Part model, mm, in its own coordinate system. Face numbers are marked on the shaded views. A direction names the side the tool comes from. Round coordinates to 2 decimals unless told otherwise and drop trailing zeros. Loops run counter-clockwise (first coordinate to the right, second up) from the corner with the lowest first, then second, coordinate; pieces in that order, holes last. Notation, with made-up numbers: (-28.5, 19.5) -> (19.5, 19.5) arc R19 ccw to (19.5, 42.5) -> close; hole circle Ø9 at (0, 19). An arc over 180 degrees is marked (long way). Use a Markdown table: item, result. Add a question column.
Item 1: Cut at D-D, the plane x = -0.5. List the corners of the cut face in (y, z).
Item 2: Cut at B-B, the plane y = 8. List the corners of the cut face in (x, z), plus the area to 3 significant figures.
Item 3: Probe line 1 (X direction, y = 2.75, z = -5.15); line 2 (Z direction, x = 11.1, y = 2); line 3 (Z direction, x = -11.1, y = 6.75). List the from-to ranges inside material, lowest first. Write a range as [from, to].
Item 4: Cut at A-A, the plane x = 11.1. List the corners of the cut face in (y, z).
Item 5: Cut at C-C, the plane z = -5.15. List the corners of the cut face in (x, y).
Item 6: Flat gauge pins, fed straight in: pin 1 (2 mm diameter, centred on x = -6.5, z = -9.5, fed in from +Y); pin 2 (1.2 mm diameter, centred on x = -6, z = -9, fed in from -Y); pin 3 (2.5 mm diameter, centred on x = 19, y = 4.5, fed in from +Z); pin 4 (5 mm diameter, centred on x = 11.1, z = -5.15, fed in from -Y). Where does each tip first touch, or does it go through?
Item 7: Which spindle directions (+Z, -Z, +X, -X, +Y, -Y) get a long thin tool onto all of the face, cutting with end or side? Do the marked faces 4, 5, 6, 7 and 8. Say none if no direction does.
Item 8: Two-plate mould, pull along Z, no slides. Class the marked faces 1, 2 and 3: pulls with the +Z half, pulls with the -Z half, needs draft (parallel to the pull), parting line crosses it, or undercut.
```python
from build123d import *

# Parameters (mm, degrees)
SKETCH_1_W          = 28
SKETCH_1_H          = 16
EXTRUDE_1_DEPTH     = 10
FILLET_1_R          = 2
SKETCH_2_R          = 1.55
CUT_EXTRUDE_1_DEPTH = 10
SKETCH_3_W          = 0.5
SKETCH_3_H          = 8
EXTRUDE_2_DEPTH     = 9
SKETCH_4_W          = 3
SKETCH_4_H          = 3
EXTRUDE_3_DEPTH     = 2.5
FILLET_2_R          = 1


with BuildPart() as part:
    # 스케치1 → 보스-돌출1 (new body)
    with BuildSketch(Plane(origin=(0, 0, 0), x_dir=(1, 0, 0), z_dir=(0, 1, 0))):
        Rectangle(SKETCH_1_W, SKETCH_1_H)
    extrude(amount=EXTRUDE_1_DEPTH)

    # 필렛1
    fillet_1_edges = [part.edges().sort_by_distance(p)[0] for p in [
        (-14, 5, -8),
        (14, 5, -8),
        (14, 5, 8),
        (-14, 5, 8),
    ]]
    fillet(fillet_1_edges, radius=FILLET_1_R)

    # 스케치2 → 컷-돌출1 (cut)
    with BuildSketch(Plane(origin=(0, 10, 0), x_dir=(1, 0, 0), z_dir=(0, 1, 0))):
        with Locations((11.1, 5.15)):
            Circle(SKETCH_2_R)
        with Locations((-11.1, -5.15)):
            Circle(SKETCH_2_R)
    extrude(amount=-CUT_EXTRUDE_1_DEPTH, mode=Mode.SUBTRACT)

    # 스케치3 → 보스-돌출2 (add)
    with BuildSketch(Plane(origin=(14, 0, 0), x_dir=(0, 0, -1), z_dir=(1, 0, 0))):
        with Locations((-2.65, 5)):
            Rectangle(SKETCH_3_W, SKETCH_3_H)
        with Locations((2.65, 5)):
            Rectangle(SKETCH_3_W, SKETCH_3_H)
    extrude(amount=EXTRUDE_2_DEPTH)

    # 스케치4 → 보스-돌출3 (add)
    with BuildSketch(Plane(origin=(0, 0, -8), x_dir=(-1, 0, 0), z_dir=(0, 0, -1))):
        with Locations((6.465564218, 5)):
            Rectangle(SKETCH_4_W, SKETCH_4_H)
    extrude(amount=EXTRUDE_3_DEPTH)

    # 필렛2
    fillet_2_edges = [part.edges().sort_by_distance(p)[0] for p in [
        (-4.965564218, 5, -10.5),
        (-7.965564218, 5, -10.5),
    ]]
    fillet(fillet_2_edges, radius=FILLET_2_R)


solid = part.part
```
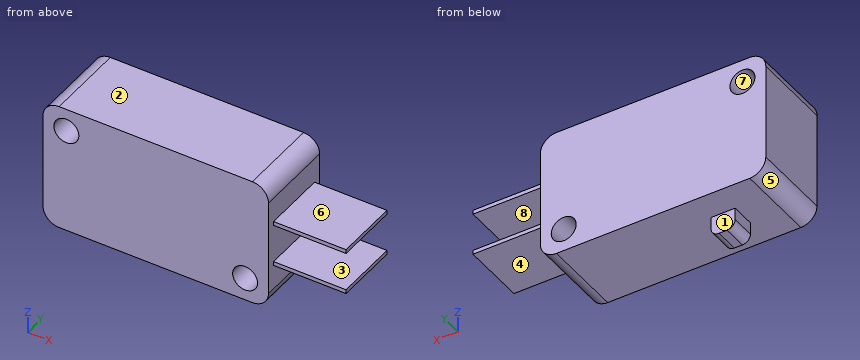
A:
| question | item | result |
|---|---|---|
| 1 | outline | (0, -8) -> (10, -8) -> (10, 8) -> (0, 8) -> close |
| 2 | outline | (-14, -6) arc R2 ccw to (-12, -8) -> (12, -8) arc R2 ccw to (14, -6) -> (14, -2.9) -> (23, -2.9) -> (23, -2.4) -> (14, -2.4) -> (14, 2.4) -> (23, 2.4) -> (23, 2.9) -> (14, 2.9) -> (14, 6) arc R2 ccw to (12, 8) -> (-12, 8) arc R2 ccw to (-14, 6) -> close; hole circle Ø3.1 at (-11.1, 5.15); hole circle Ø3.1 at (11.1, -5.15) |
| 2 | area | 438 mm^2 |
| 3 | line 1 | x = [-14, 9.55], [12.65, 14] |
| 3 | line 2 | z = [-8, -6.7], [-3.6, 8] |
| 3 | line 3 | z = [-8, 3.6], [6.7, 8] |
| 4 | outline | (0, -8) -> (10, -8) -> (10, -6.7) -> (0, -6.7) -> close; (0, -3.6) -> (10, -3.6) -> (10, 8) -> (0, 8) -> close |
| 5 | outline | (-14, 0) -> (9.55, 0) -> (9.55, 10) -> (-14, 10) -> close; (12.65, 0) -> (14, 0) -> (14, 10) -> (12.65, 10) -> close |
| 6 | pin 1 | stops at y = 6.5 |
| 6 | pin 2 | stops at y = 3.5 |
| 6 | pin 3 | stops at z = 2.9 |
| 6 | pin 4 | stops at y = 0 |
| 7 | face 4 | -Z, +X, +Y, -Y |
| 7 | face 5 | -Z, -X, +Y, -Y |
| 7 | face 6 | +Z, +X, +Y, -Y |
| 7 | face 7 | +Y, -Y |
| 7 | face 8 | +X, +Y, -Y |
| 8 | face 1 | needs draft |
| 8 | face 2 | pulls with the +Z half |
| 8 | face 3 | undercut |
